Source: CAD feature listing. Evaluate the final solid. Frame: model axes, mm. A direction names the side the tool comes from. Give positions to 0.01 mm unless a question says otherwise; leave off trailing zeros. Order: outer loops, then holes, each group sorted by start corner. A loop starts at its lowest first (then second) coordinate and runs counter-clockwise, first axis right, second up. Notation, with made-up numbers: M 58.25,51 L 63.25,51 A17 cw 63.25,81 Z; hole C 50.25,47.25 d6. An arc over 180 degrees is marked long. One line per question, with ' | ' between items. Start each with the question number.
from build123d import *

# Parameters (mm, degrees)
ESQUISSE1_R                  = 16.5
ESQUISSE1_R_2                = 14
BOSS_EXTRU_1_DEPTH           = 10
ESQUISSE2_R                  = 16.5
BOSS_EXTRU_2_DEPTH           = 3
CHANFREIN1_SIZE              = 1
ENL_V_MAT_EXTRU_1_DEPTH      = 27.711420778
ENL_V_MAT_EXTRU_1_DEPTH_BACK = 27.711420778
ESQUISSE3_R                  = 4.1
CHANFREIN2_SIZE              = 1


with BuildPart() as part:
    # Esquisse1 → Boss.-Extru.1 (new body)
    with BuildSketch(Plane.XY):
        Circle(ESQUISSE1_R)
        Circle(ESQUISSE1_R_2, mode=Mode.SUBTRACT)
    extrude(amount=BOSS_EXTRU_1_DEPTH)

    # Esquisse2 → Boss.-Extru.2 (add)
    with BuildSketch(Plane.XY.offset(10)):
        Circle(ESQUISSE2_R)
    extrude(amount=BOSS_EXTRU_2_DEPTH)

    # Chanfrein1
    chanfrein1_edges = [part.edges().sort_by_distance(p)[0] for p in [
        (-14, 0, 0),
    ]]
    chamfer(chanfrein1_edges, length=CHANFREIN1_SIZE)

    # Esquisse3 → Enlèv. mat.-Extru.1 (cut, two sides: drawn at the far end of the back side and taken through both)
    with BuildSketch(Plane.XY.offset(13).offset(-ENL_V_MAT_EXTRU_1_DEPTH_BACK)):
        Circle(ESQUISSE3_R)
    extrude(amount=ENL_V_MAT_EXTRU_1_DEPTH + ENL_V_MAT_EXTRU_1_DEPTH_BACK, mode=Mode.SUBTRACT)

    # Chanfrein2
    chanfrein2_edges = [part.edges().sort_by_distance(p)[0] for p in [
        (-16.5, 0, 13),
    ]]
    chamfer(chanfrein2_edges, length=CHANFREIN2_SIZE)


solid = part.part
Item 1: Cut plane A-A on y = 0. Return the cut outline in (x, z), and give its area (3 significant figures).
Item 2: Cut plane C-C on z = 8.5. Return the cut outline in (x, y).
Item 3: Mould query, pull axis X, two halves, no side actions, for faces 3 (the flat face through (2.9, 3.3, 10)), 4 (the flat face through (4, -15, 0)), 5 (the cylindrical face through (15.24, -6.32, 5.92)). Classes: pulls with the +X half, pulls with the -X half, needs draft (parallel to the pull), parting line crosses it, or undercut.
Item 4: Line query: line 1 (Y direction, x = 0, z = 5.25); line 2 (Y direction, x = 0, z = 11.15); line 3 (Z direction, x = 9.5, y = -6.5). Output: solid intervals per line, ascending.
Item 5: Reachability of faces 1 (the cylindrical face through (-0.534, 4.065, 11.479)), 2 (the cylindrical face through (12.932, -5.362, 5.437)) from +Z, -Z, +X, -X, +Y, -Y: full face, straight path, thin tool, end or side. Return the list, or none.
Item 6: Pin query (flat end, axial travel): pin 1 Ø3 at (x, z) = (-9, 3) entering from -Y; pin 2 Ø6 at (x, z) = (7.5, 5.5) entering from +Y; pin 3 Ø14 at (x, y) = (4.5, 3.5) entering from -Z. Return the tip coordinate at first contact, or that it passes through.
Results are:
1) outline: M -16.5,0 L -15,0 L -14,1 L -14,10 L -4.1,10 L -4.1,13 L -15.5,13 L -16.5,12 Z; M 4.1,10 L 14,10 L 14,1 L 15,0 L 16.5,0 L 16.5,12 L 15.5,13 L 4.1,13 Z | area: 122 mm2
2) outline: C 0,0 d33; hole C 0,0 d28
3) face 3: undercut | face 4: needs draft | face 5: parting line crosses it
4) line 1: y = -16.5 to -14, 14 to 16.5 | line 2: y = -16.5 to -4.1, 4.1 to 16.5 | line 3: z = 10 to 13
5) face 1: +Z, -Z | face 2: -Z
6) pin 1: stops at y = -14.7 | pin 2: stops at y = 15.87 | pin 3: stops at z = 10
